```python
from build123d import *

# Parameters (mm, degrees)
SKETCH_1_W      = 2.9999
SKETCH_1_H      = 9.999
EXTRUDE_1_DEPTH = 3


with BuildPart() as part:
    # 草图1 → 凸台-拉伸1 (new body)
    with BuildSketch(Plane.XY.offset(3)):
        Polygon((42.580009157, 5.99999), (42.580009157, 7.99949), (38.581009157, 7.99949), (38.581009157, 6.74959), (36.079809157, 6.74959), (36.079809157, 7.99949), (31.580009157, 7.99949), (31.580009157, 10.99949), (36.079809157, 10.99949), (36.079809157, 12.25079), (38.581009157, 12.25079), (38.581009157, 10.99949), (42.580009157, 10.99949), (42.580009157, 13.00039), (45.579909157, 13.00039), (45.579909157, 19.000390002), (-4.419390843, 19.000390002), (-4.419390843, 13.00039), (-1.419350843, 13.00039), (-1.419350843, 10.99949), (2.579649157, 10.99949), (2.579649157, 12.25079), (5.080849157, 12.25079), (5.080849157, 10.99949), (9.580649157, 10.99949), (9.580649157, 7.99949), (5.080849157, 7.99949), (5.080849157, 6.74959), (2.579649157, 6.74959), (2.579649157, 7.99949), (-1.419350843, 7.99949), (-1.419350843, 5.99999), (-4.419250843, 5.99999), (-4.419250843, -2e-09), (45.580189157, -2e-09), (45.580189157, 5.99999), align=None)
        with Locations((17.580299157, 9.50019)):
            Rectangle(SKETCH_1_W, SKETCH_1_H, mode=Mode.SUBTRACT)
    extrude(amount=-EXTRUDE_1_DEPTH)


solid = part.part
```
Geometry: final body of the model. Coordinates: model frame, mm. A direction names the side the tool comes from. Round coordinates to 2 decimals unless told otherwise and drop trailing zeros. Write each loop counter-clockwise with the first axis right and the second up, starting at its lowest first coordinate (ties: lowest second). Pieces come first, ordered by that corner, then holes. Notation, with made-up numbers: (-24.5, 53) -> (-10.5, 53) arc R13 cw to (-10.5, 69) -> close; hole circle Ø9 at (52, 37.25). An arc over 180 degrees is marked (long way). Return JSON: item names as keys, results as strings.
Q1. Ray query, line 1 (X direction, y = 13.75, z = 2.6); line 2 (Y direction, x = 2, z = 0.95); line 3 (Y direction, x = 18.5, z = 0.4). Return the intervals inside material, ascending.
From the geometry:
{"line 1": "-4.42 to 16.08, 19.08 to 45.58", "line 2": "0 to 8, 11 to 19", "line 3": "0 to 4.5, 14.5 to 19"}
Q2. First-contact query: pin 1 Ø1 at (y, z) = (12, 1.5) entering from -X; pin 2 Ø1.4 at (y, z) = (7, 1) entering from +X. Flat tips, straight axial feed; report the tip coordinate or a pass-through.
From the geometry:
{"pin 1": "x = -1.42", "pin 2": "x = 42.58"}
Q3. Section B-B on x = 33. Return the cut outline in (y, z).
From the geometry:
{"outline": "(0, 0) -> (8, 0) -> (8, 3) -> (0, 3) -> close; (11, 0) -> (19, 0) -> (19, 3) -> (11, 3) -> close"}
Q4. Mould query, pull axis X, two halves, no side actions, for faces 1 (the flat face through (-1.419, 7, 2)), 2 (the flat face through (42.58, 12, 2)), 3 (the flat face through (38.581, 7, 2)), 4 (the flat face through (2.58, 12, 2)). Classes: +X half, -X half, draft (parallel to the pull), parting line (faces both ways), or undercut.
From the geometry:
{"face 1": "-X half", "face 2": "+X half", "face 3": "undercut", "face 4": "undercut"}
Q5. Section A-A on y = 13.5. Return the cut outline in (x, z), and give its area (3 significant figures).
From the geometry:
{"outline": "(-4.42, 0) -> (16.08, 0) -> (16.08, 3) -> (-4.42, 3) -> close; (19.08, 0) -> (45.58, 0) -> (45.58, 3) -> (19.08, 3) -> close", "area": "141 mm2"}
Q6. Set-up query: faces 5 (the flat face through (1, 7.999, 2)), 6 (the flat face through (44, 6, 2)), 7 (the flat face through (2.58, 7, 2)). Return all of +Z, -Z, +X, -X, +Y, -Y with unobstructed straight access to the full face (end or side cutting, diameter ignored); none if empty.
From the geometry:
{"face 5": "+Z, -Z, -X", "face 6": "+Z, -Z, +X", "face 7": "+Z, -Z"}
